Answer from the drawing. Dimensions are ordinates in mm from the lowest x, y and z of the part. A direction names the side the tool comes from. Coordinates: 2 decimals unless noted, no trailing zeros. Order: outer loops, then holes, each group sorted by start corner. A loop starts at its lowest first (then second) coordinate and runs counter-clockwise, first axis right, second up. Notation, with made-up numbers: (58.5, -21) - (63.5, -21) arc R13 ccw to (63.5, 3) - close; hole circle Ø11 at (60.5, -13.5). An arc over 180 degrees is marked (long way). Answer as a JSON object with one key per item and string values. Group by question number.
1) Section C-C (y = 137.5) is taken. Give the vertices of the cut face in (x, z) (3 decimals), plus the area to 3 significant figures.
2) Section A-A (x = 99) is taken. Give the vertices of the cut face in (y, z) (3 decimals).
3) Find the intervals of material crossed by line 1 along Y through (x, z) = (179.5, 20.75) (3 decimals); line 2 along X through (y, z) = (144.5, 20); line 3 along X through (y, z) = (110, 10), in increasing order.
4) A tool of negligible diameter and unlimited length cuts with its end or side. For the marked faces 1, 2 and 3, from which of +Z, -Z, +X, -X, +Y, -Y can it reach the whole face along a straight path? Write none if from no direction.
5) The mould has two halves that part along X. Classify the marked faces 4, 5 and 6: released by +X, released by -X, zero draft, split by the parting line, or undercut.
6) Section B-B (z = 10) is taken. Give the vertices of the cut face in (x, y) (3 decimals).
7) This flat-tipped pin is pushed along its axis until it touches: P1, Ø1.5, axis at x = 205, z = 13, coming from the -Y side. Where does it stop, or does it pass through?
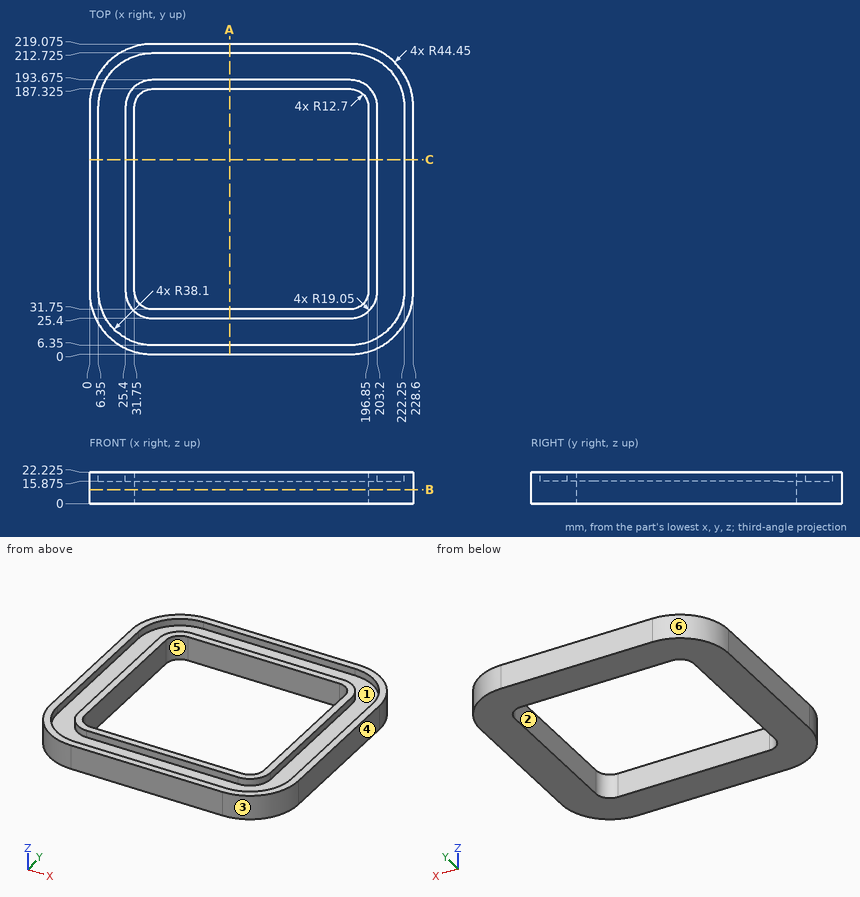
Report:
{
 "1": {"outline": "(0, 0) - (31.75, 0) - (31.75, 22.225) - (25.4, 22.225) - (25.4, 15.875) - (6.35, 15.875) - (6.35, 22.225) - (0, 22.225) - close; (196.85, 0) - (228.6, 0) - (228.6, 22.225) - (222.25, 22.225) - (222.25, 15.875) - (203.2, 15.875) - (203.2, 22.225) - (196.85, 22.225) - close", "area": "1,170 mm²"},
 "2": {"outline": "(0, 0) - (31.75, 0) - (31.75, 22.225) - (25.4, 22.225) - (25.4, 15.875) - (6.35, 15.875) - (6.35, 22.225) - (0, 22.225) - close; (187.325, 0) - (219.075, 0) - (219.075, 22.225) - (212.725, 22.225) - (212.725, 15.875) - (193.675, 15.875) - (193.675, 22.225) - (187.325, 22.225) - close"},
 "3": {"line 1": "y = 0 to 6.35, 25.4 to 31.75, 187.325 to 193.675, 212.725 to 219.075", "line 2": "x = 0 to 6.35, 25.4 to 31.75, 196.85 to 203.2, 222.25 to 228.6", "line 3": "x = 0 to 31.75, 196.85 to 228.6"},
 "4": {"face 1": "+Z", "face 2": "+Z, -Z", "face 3": "+Z, -Z, +X, -Y"},
 "5": {"face 4": "released by +X", "face 5": "undercut", "face 6": "released by -X"},
 "6": {"outline": "(0, 44.45) arc R44.45 ccw to (44.45, 0) - (184.15, 0) arc R44.45 ccw to (228.6, 44.45) - (228.6, 174.625) arc R44.45 ccw to (184.15, 219.075) - (44.45, 219.075) arc R44.45 ccw to (0, 174.625) - close; hole (31.75, 44.45) arc R12.7 ccw to (44.45, 31.75) - (184.15, 31.75) arc R12.7 ccw to (196.85, 44.45) - (196.85, 174.625) arc R12.7 ccw to (184.15, 187.325) - (44.45, 187.325) arc R12.7 ccw to (31.75, 174.625) - close"},
 "7": {"P1": "stops at y = 4.8"}
}
